For this review, use the dimensioned drawing (mm, ordinates from the lowest corner) and the shaded views. Coordinates: 2 decimals unless noted, no trailing zeros. Loops run counter-clockwise (first coordinate to the right, second up) from the corner with the lowest first, then second, coordinate; pieces in that order, holes last. Notation, with made-up numbers: (73.25, -18) - (122.25, -18) arc R11 cw to (122.25, -10) - close; hole circle Ø11 at (7, 53). An arc over 180 degrees is marked (long way). Answer in a Markdown table with one row per item. Add a question column.
(1) We need section D-D, the plane z = 72. Write out the cut boundary in (x, y).
(2) Clearance check with flat-ended pins moving along their axes: pin 1 (1.5 mm diameter, centred on x = 1.5, z = 33.5, fed in from +Y); pin 2 (0.9 mm diameter, centred on x = 1.5, y = 59.5, fed in from -Z). State where each tip first meets the part, or that it passes through.
(3) To check wall thickness, follow L1, parallel to Y at x = 1.5, z = 72; L2, parallel to Y at x = 0.8, z = 11; L3, parallel to Z at x = 1.45, y = 33.5. State the ranges of each line that lie inside material, in increasing order. Write a range as [from, to].
(4) We need section B-B, the plane y = 13. Write out the cut boundary in (x, z).
(5) We need section A-A, the plane z = 41. Write out the cut boundary in (x, y), plus the area to 3 significant figures.
(6) We need section C-C, the plane y = 74. Write out the cut boundary in (x, z).
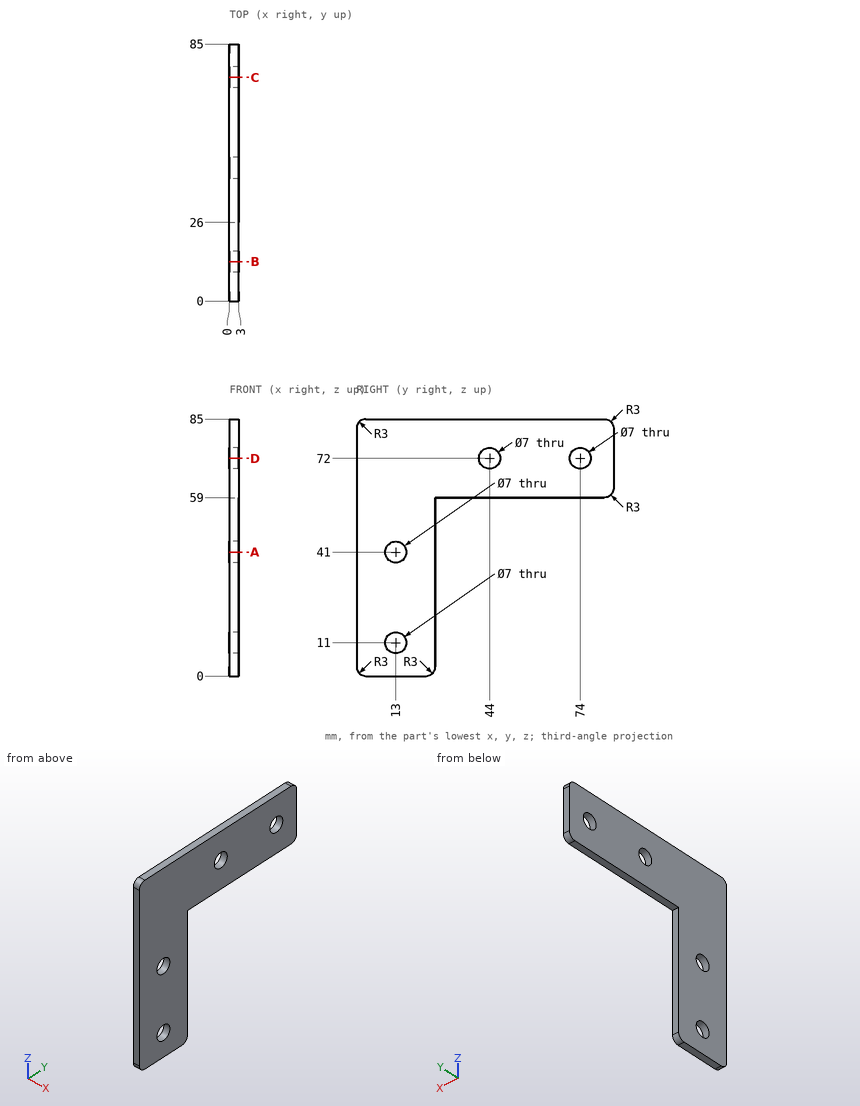
Responses:
| question | item | result |
|---|---|---|
| 1 | outline | (0, 0) - (3, 0) - (3, 40.5) - (0, 40.5) - close; (0, 47.5) - (3, 47.5) - (3, 70.5) - (0, 70.5) - close; (0, 77.5) - (3, 77.5) - (3, 85) - (0, 85) - close |
| 2 | pin 1 | stops at y = 26 |
| 2 | pin 2 | stops at z = 59 |
| 3 | L1 | y = [0, 40.5], [47.5, 70.5], [77.5, 85] |
| 3 | L2 | y = [0, 9.5], [16.5, 26] |
| 3 | L3 | z = [59, 85] |
| 4 | outline | (0, 0) - (3, 0) - (3, 7.5) - (0, 7.5) - close; (0, 14.5) - (3, 14.5) - (3, 37.5) - (0, 37.5) - close; (0, 44.5) - (3, 44.5) - (3, 85) - (0, 85) - close |
| 5 | outline | (0, 0) - (3, 0) - (3, 9.5) - (0, 9.5) - close; (0, 16.5) - (3, 16.5) - (3, 26) - (0, 26) - close |
| 5 | area | 57.0 mm2 |
| 6 | outline | (0, 59) - (3, 59) - (3, 68.5) - (0, 68.5) - close; (0, 75.5) - (3, 75.5) - (3, 85) - (0, 85) - close |
